```python
from build123d import *

# Parameters (mm, degrees)
SALIENTE_EXTRUIR1_DEPTH      = 6.5024
SALIENTE_EXTRUIR1_DEPTH_BACK = 6.5024
SALIENTE_EXTRUIR2_DEPTH      = 5.0038
SALIENTE_EXTRUIR2_DEPTH_BACK = 5.0038
CROQUIS1_4_W                 = 5.9944
CROQUIS1_4_H                 = 3.9878
SALIENTE_EXTRUIR3_DEPTH      = 3.4671
SALIENTE_EXTRUIR3_DEPTH_BACK = 3.4671
CROQUIS2_W                   = 5.0038
CROQUIS2_H                   = 0.508
CROQUIS2_H_2                 = 1.524
CROQUIS2_W_2                 = 1.4986
CROQUIS2_H_3                 = 10.4902
CORTAR_EXTRUIR1_DEPTH        = 0.508
CROQUIS3_OUTSIDE_W           = 20.026
CROQUIS3_OUTSIDE_H           = 23.024
CORTAR_EXTRUIR2_DEPTH        = 3.9878
CORTAR_EXTRUIR3_DEPTH        = 3.9878


with BuildPart() as part:
    # Croquis1 → Saliente-Extruir1 (new body, two sides)
    with BuildSketch(Plane(origin=(0, 0, 0), x_dir=(0, 0, -1), z_dir=(1, 0, 0))) as saliente_extruir1_sk:
        Polygon((-3.5052, 3.0099), (-7.493, 3.0099), (-8.001, 3.0099), (-8.001, 2.5019), (-7.0104, 2.5019), (-7.0104, -2.5019), (7.0104, -2.5019), (7.0104, 2.5019), (8.001, 2.5019), (8.001, 3.0099), (6.477, 3.0099), align=None)
    extrude(amount=SALIENTE_EXTRUIR1_DEPTH)
    extrude(saliente_extruir1_sk.sketch, amount=-SALIENTE_EXTRUIR1_DEPTH_BACK)

    # Croquis1<3> → Saliente-Extruir2 (add, two sides)
    with BuildSketch(Plane(origin=(0, 0, 0), x_dir=(0, 0, -1), z_dir=(1, 0, 0))) as saliente_extruir2_sk:
        with BuildLine():
            Line((-2.868527833, 7.8359), (-3.376527833, 7.8359))
            Line((-3.376527833, 7.8359), (-7.493, 3.0099))
            Line((-7.493, 3.0099), (-3.5052, 3.0099))
            Line((-3.5052, 3.0099), (6.477, 3.0099))
            Line((6.477, 3.0099), (4.937272491, 7.021027296))
            ThreePointArc((4.937272491, 7.021027296), (4.47096127, 7.61254026), (3.751625349, 7.8359))
            Line((3.751625349, 7.8359), (3.125872167, 7.8359))
            Line((3.125872167, 7.8359), (-2.868527833, 7.8359))
        make_face()
    extrude(amount=SALIENTE_EXTRUIR2_DEPTH)
    extrude(saliente_extruir2_sk.sketch, amount=-SALIENTE_EXTRUIR2_DEPTH_BACK)

    # Croquis1<4> → Saliente-Extruir3 (add, two sides)
    with BuildSketch(Plane(origin=(0, 0, 0), x_dir=(0, 0, -1), z_dir=(1, 0, 0))) as saliente_extruir3_sk:
        with Locations((0.128672167, 9.8298)):
            Rectangle(CROQUIS1_4_W, CROQUIS1_4_H)
    extrude(amount=SALIENTE_EXTRUIR3_DEPTH)
    extrude(saliente_extruir3_sk.sketch, amount=-SALIENTE_EXTRUIR3_DEPTH_BACK)

    # Croquis2 → Cortar-Extruir1 (cut)
    with BuildSketch(Plane(origin=(0, 3.0099, 0), x_dir=(1, 0, 0), z_dir=(0, 1, 0))):
        with Locations((0, -7.747)):
            Rectangle(CROQUIS2_W, CROQUIS2_H)
        with Locations((0, 7.239)):
            Rectangle(CROQUIS2_W, CROQUIS2_H_2)
        with Locations((-5.7531, 0)):
            Rectangle(CROQUIS2_W_2, CROQUIS2_H_3)
        with Locations((5.7531, 0)):
            Rectangle(CROQUIS2_W_2, CROQUIS2_H_3)
    extrude(amount=-CORTAR_EXTRUIR1_DEPTH, mode=Mode.SUBTRACT)

    # Croquis3 outside → Cortar-Extruir2 (cut)
    with BuildSketch(Plane(origin=(0, 11.8237, 0), x_dir=(1, 0, 0), z_dir=(0, 1, 0))):
        Rectangle(CROQUIS3_OUTSIDE_W, CROQUIS3_OUTSIDE_H)
        Polygon((-3.4671, 3.125872167), (-3.4671, -2.868527833), (-1.9685, -2.868527833), (-1.9685, -2.614527833), (-3.2131, -2.614527833), (-3.2131, 2.871872167), (-1.9685, 2.871872167), (-1.9685, 3.125872167), align=None, mode=Mode.SUBTRACT)
        Polygon((0.508, 1.9685), (-0.508, 1.9685), (-0.508, 0.508), (-1.9685, 0.508), (-1.9685, -0.508), (-0.508, -0.508), (-0.508, -1.9685), (0.508, -1.9685), (0.508, -0.508), (1.9685, -0.508), (1.9685, 0.508), (0.508, 0.508), align=None, mode=Mode.SUBTRACT)
        Polygon((3.2131, 2.871872167), (3.2131, -2.614527833), (1.9685, -2.614527833), (1.9685, -2.868527833), (3.4671, -2.868527833), (3.4671, 3.125872167), (1.9685, 3.125872167), (1.9685, 2.871872167), align=None, mode=Mode.SUBTRACT)
    extrude(amount=-CORTAR_EXTRUIR2_DEPTH, mode=Mode.SUBTRACT)

    # Croquis3<2> → Cortar-Extruir3 (cut)
    with BuildSketch(Plane(origin=(0, 11.8237, 0), x_dir=(1, 0, 0), z_dir=(0, 1, 0))):
        Polygon((-3.4671, 3.125872167), (-3.4671, -2.868527833), (-1.9685, -2.868527833), (-1.9685, -2.614527833), (-3.2131, -2.614527833), (-3.2131, 2.871872167), (-1.9685, 2.871872167), (-1.9685, 3.125872167), align=None)
        Polygon((3.2131, 2.871872167), (3.2131, -2.614527833), (1.9685, -2.614527833), (1.9685, -2.868527833), (3.4671, -2.868527833), (3.4671, 3.125872167), (1.9685, 3.125872167), (1.9685, 2.871872167), align=None)
    extrude(amount=-CORTAR_EXTRUIR3_DEPTH, mode=Mode.SUBTRACT)


solid = part.part
```
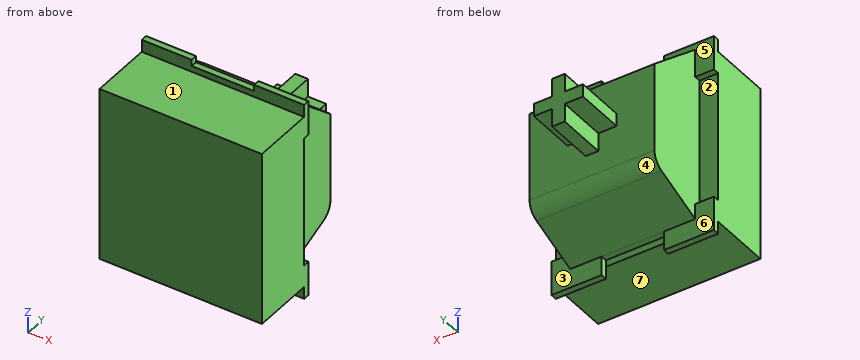
CAD build for the part. Positions are in the model's coordinates, mm. Face numbers are marked on the shaded views. A direction names the side the tool comes from. Give positions to 0.01 mm unless a question says otherwise; leave off trailing zeros. Write each loop counter-clockwise with the first axis right and the second up, starting at its lowest first coordinate (ties: lowest second). Pieces come first, ordered by that corner, then holes. Notation, with made-up numbers: M 32.25,27.5 L 74.25,27.5 A11 cw 74.25,45.5 Z; hole C 85.25,-1.5 d11. An arc over 180 degrees is marked long. Return JSON: item names as keys, results as strings. Group by question number.
(1) Drill centre lines: L1, parallel to Y at x = 5.75, z = -6; L2, parallel to Y at x = -2.5, z = 2.25; L3, parallel to X at y = 4.25, z = -5. Where is each one in solid material? Low to high. Write a range as [from, to].
(2) Band-saw the part on D-D (x = -0.25). Give the cut face in (y, z), and give its area (3 significant figures).
(3) Band-saw the part on A-A (y = 10). Give the cut face in (x, z), and give its area (3 significant figures).
(4) Flat gauge pins, fed straight in: pin 1 Ø6 at (x, y) = (-1.5, 8) entering from +Z; pin 2 Ø1.2 at (x, y) = (-1.5, 10.5) entering from -Z; pin 3 Ø1.5 at (x, y) = (-0.5, 1) entering from +Z. Where does each tip first touch, or does it go through?
(5) Band-saw the part on C-C (z = 1). Give the cut face in (x, y).
(6) Mould opens along Z. For the marked faces 1, 2, 3 and 4 say: pulls with the +Z half, pulls with the -Z half, needs draft (parallel to the pull), parting line crosses it, or undercut.
(7) Band-saw the part on B-B (x = 4.5). Give the cut face in (y, z), and give its area (3 significant figures).
(8) 3-axis set-ups, long thin cutter, end or side, ignore diameter. For the marked faces 5, 6 and 7: which of +Z, -Z, +X, -X, +Y, -Y reach the whole face in a straight line?
Entries:
{
 "1": {"L1": "y = [-2.5, 3.01]", "L2": "y = [-2.5, 7.84]", "L3": "x = [-5, 5]"},
 "2": {"outline": "M -2.5,-7.01 L 2.5,-7.01 L 2.5,-6.48 L 3.01,-6.48 L 7.02,-4.94 A1.27 ccw 7.84,-3.75 L 7.84,-1.97 L 11.82,-1.97 L 11.82,1.97 L 7.84,1.97 L 7.84,3.38 L 3.01,7.49 L 2.5,7.49 L 2.5,7.01 L -2.5,7.01 Z", "area": "146 mm^2"},
 "3": {"outline": "M -1.97,-0.51 L -0.51,-0.51 L -0.51,-1.97 L 0.51,-1.97 L 0.51,-0.51 L 1.97,-0.51 L 1.97,0.51 L 0.51,0.51 L 0.51,1.97 L -0.51,1.97 L -0.51,0.51 L -1.97,0.51 Z", "area": "6.97 mm^2"},
 "4": {"pin 1": "stops at z = 5.8", "pin 2": "stops at z = -0.51", "pin 3": "stops at z = 7.01"},
 "5": {"outline": "M -6.5,-2.5 L 6.5,-2.5 L 6.5,2.5 L 5,2.5 L 5,7.84 L 0.51,7.84 L 0.51,11.82 L -0.51,11.82 L -0.51,7.84 L -5,7.84 L -5,2.5 L -6.5,2.5 Z"},
 "6": {"face 1": "pulls with the +Z half", "face 2": "undercut", "face 3": "needs draft", "face 4": "pulls with the -Z half"},
 "7": {"outline": "M -2.5,-7.01 L 2.5,-7.01 L 2.5,-8 L 3.01,-8 L 3.01,-6.48 L 7.02,-4.94 A1.27 ccw 7.84,-3.75 L 7.84,3.38 L 3.01,7.49 L 3.01,8 L 2.5,8 L 2.5,7.01 L -2.5,7.01 Z", "area": "131 mm^2"},
 "8": {"face 5": "+Z, -X, +Y", "face 6": "-Z, -X, +Y", "face 7": "-Z, +X, -X, -Y"}
}
